Geometry: final body of the model. Coordinates: model frame, mm. Coordinates: 2 decimals unless noted, no trailing zeros. Write each loop counter-clockwise with the first axis right and the second up, starting at its lowest first coordinate (ties: lowest second). Pieces come first, ordered by that corner, then holes. Notation, with made-up numbers: (16.5, 17.25) - (54.5, 17.25) arc R19 cw to (54.5, 47.25) - close; hole circle Ø8 at (-35, 63.25). An arc over 180 degrees is marked (long way). Answer as a JSON object with one key per item and string values. Group by question number.
Item 1: Line query: line 1 along X through (y, z) = (114, -0.4); line 2 along Y through (x, z) = (85, 0.5). Output: solid intervals per line, ascending. Write a range as from..to.
Item 2: Section A-A on x = 62.5. Return loops of the section in (y, z), and give its area (3 significant figures).
Item 3: Section B-B on z = 0.5. Return loops of the section in (x, y), and give its area (3 significant figures).
Autodesk Inventor part; units mm, degrees
ref_plane "YZ Plane" through (0, 0, 0) normal (1, 0, 0) x (0, 1, 0)
ref_plane "XZ Plane" through (0, 0, 0) normal (0, 1, 0) x (-1, 0, 0)
ref_plane "XY Plane" through (0, 0, 0) normal (0, 0, 1) x (1, 0, 0)
sketch "Sketch1" plane through (0, 0, 0) normal (0, 0, 1) x (1, 0, 0)
  line L0 (-584, -184) -> (584, -184)
  line L1 (584, -184) -> (584, 184)
  line L2 (584, 184) -> (-584, 184)
  line L3 (-584, 184) -> (-584, -184)
  line L4 (-584, -184) -> (584, 184) construction
  line L5 (584, -184) -> (-584, 184) construction
  line L6 (-550, 159) -> (-350, 159)
  line L7 (-350, 159) -> (-350, 84)
  line L8 (-350, 84) -> (-550, 84)
  line L9 (-550, 84) -> (-550, 159)
  line L10 (-325, 84) -> (-325, 159)
  line L11 (-325, 159) -> (-125, 159)
  line L12 (-125, 159) -> (-125, 84)
  line L13 (-125, 84) -> (-325, 84)
  line L14 (-100, 84) -> (-100, 159)
  line L15 (-100, 159) -> (100, 159)
  line L16 (100, 159) -> (100, 84)
  line L17 (100, 84) -> (-100, 84)
  line L18 (125, 84) -> (125, 159)
  line L19 (125, 159) -> (325, 159)
  line L20 (325, 159) -> (325, 84)
  line L21 (325, 84) -> (125, 84)
  line L22 (350, 84) -> (350, 159)
  line L23 (350, 159) -> (550, 159)
  line L24 (550, 159) -> (550, 84)
  line L25 (550, 84) -> (350, 84)
  point P0 (0, 0)
  point P1 (-550, 121.5)
  point P2 (-325, 121.5)
  point P3 (-100, 121.5)
  point P4 (125, 121.5)
  point P5 (350, 121.5)
  dimension "d0" = 1168
  dimension "d1" = 368
  dimension "d2" = 75
  dimension "d3" = 25
  dimension "d4" = 200
  dimension "d5" = 34
  dimension "d10" = 225
extrude "Extrusion2" add sketch "Sketch1" along normal mid plane 3
properties part number "Lado" material "Acrylic"
Checks:
{
 "1": {"line 1": "-584..-550, -350..-325, -125..-100, 100..125, 325..350, 550..584", "line 2": "-184..84, 159..184"},
 "2": {"outline": "(-184, -1.5) - (84, -1.5) - (84, 1.5) - (-184, 1.5) - close; (159, -1.5) - (184, -1.5) - (184, 1.5) - (159, 1.5) - close", "area": "879 mm^2"},
 "3": {"outline": "(-584, -184) - (584, -184) - (584, 184) - (-584, 184) - close; hole (-550, 84) - (-350, 84) - (-350, 159) - (-550, 159) - close; hole (-325, 84) - (-125, 84) - (-125, 159) - (-325, 159) - close; hole (-100, 84) - (100, 84) - (100, 159) - (-100, 159) - close; hole (125, 84) - (325, 84) - (325, 159) - (125, 159) - close; hole (350, 84) - (550, 84) - (550, 159) - (350, 159) - close", "area": "355,000 mm^2"}
}
